```python
from build123d import *

# Parameters (mm, degrees)
SKETCH1_R                               = 75
BOSS_EXTRUDE1_DEPTH                     = 10
SKETCH3_R                               = 4.5
CUT_EXTRUDE2_DEPTH                      = 10
SKETCH5_W                               = 2.667
SKETCH5_H                               = 4.572
SKETCH6_R                               = 55
SKETCH6_R_2                             = 53
CUT_EXTRUDE3_DEPTH                      = 1.3208
SKETCH10_R                              = 2
CUT_EXTRUDE6_DEPTH                      = 11
CBORE_FOR_M5_HEX_HEAD_BOLT1_D           = 5.5
CBORE_FOR_M5_HEX_HEAD_BOLT1_CBORE_D     = 12.238
CBORE_FOR_M5_HEX_HEAD_BOLT1_CBORE_DEPTH = 3.5
SKETCH16_R                              = 75
SKETCH16_R_2                            = 68
CUT_EXTRUDE10_DEPTH                     = 10
CIRPATTERN1_COUNT                       = 12
CIRPATTERN2_COUNT                       = 8
SKETCH17_R                              = 6.119
CUT_EXTRUDE11_DEPTH                     = 5
CIRPATTERN3_COUNT                       = 8
SKETCH18_R                              = 15
CUT_EXTRUDE12_DEPTH                     = 10


with BuildPart() as part:
    # Sketch1 → Boss-Extrude1 (new body)
    with BuildSketch(Plane.XY):
        Circle(SKETCH1_R)
    extrude(amount=BOSS_EXTRUDE1_DEPTH)

    # Sketch3 → Cut-Extrude2 (cut)
    with BuildSketch(Plane.XY.offset(10)):
        Circle(SKETCH3_R)
    extrude(amount=-CUT_EXTRUDE2_DEPTH, mode=Mode.SUBTRACT)

    # Sketch5 → Cut-Revolve1 (revolve, cut)
    with BuildSketch(Plane(origin=(0, 0, 0), x_dir=(0, 0, -1), z_dir=(1, 0, 0))):
        with Locations((-1.3335, 24.8666)):
            Rectangle(SKETCH5_W, SKETCH5_H)
    revolve(axis=Axis((0, 0, 0), (0, 0, -1)), mode=Mode.SUBTRACT)

    # Sketch6 → Cut-Extrude3 (cut)
    with BuildSketch(Plane.XY.offset(10)):
        Circle(SKETCH6_R)
        Circle(SKETCH6_R_2, mode=Mode.SUBTRACT)
    extrude(amount=-CUT_EXTRUDE3_DEPTH, mode=Mode.SUBTRACT)

    # Sketch10 → Cut-Extrude6 (cut, through all)
    with BuildSketch(Plane(origin=(0, 0, 0), x_dir=(-1, 0, 0), z_dir=(0, 0, -1))):
        with Locations((0, 61)):
            Circle(SKETCH10_R)
    cut_extrude6 = extrude(amount=-CUT_EXTRUDE6_DEPTH, mode=Mode.SUBTRACT)

    # CBORE for M5 Hex Head Bolt1 (through all)
    with Locations(Plane(origin=(0, 0, 0), x_dir=(-1, 0, 0), z_dir=(0, 0, -1))):
        with Locations((-28.284271247, 28.284271247)):
            cbore_for_m5_hex_head_bolt1 = CounterBoreHole(CBORE_FOR_M5_HEX_HEAD_BOLT1_D / 2, CBORE_FOR_M5_HEX_HEAD_BOLT1_CBORE_D / 2, CBORE_FOR_M5_HEX_HEAD_BOLT1_CBORE_DEPTH)

    # Sketch16 → Cut-Extrude10 (cut)
    with BuildSketch(Plane(origin=(0, 0, 0), x_dir=(-1, 0, 0), z_dir=(0, 0, -1))):
        Circle(SKETCH16_R)
        Circle(SKETCH16_R_2, mode=Mode.SUBTRACT)
    extrude(amount=-CUT_EXTRUDE10_DEPTH, mode=Mode.SUBTRACT)

    # CirPattern1: Cut-Extrude6 ×12 about axis
    cirpattern1_axis = Axis((0, 0, 0), (0, 0, 1))
    for i in range(1, CIRPATTERN1_COUNT):
        add(cut_extrude6.rotate(cirpattern1_axis, i * 360 / CIRPATTERN1_COUNT), mode=Mode.SUBTRACT)

    # CirPattern2: CBORE for M5 Hex Head Bolt1 ×8 about axis
    cirpattern2_axis = Axis((0, 0, 0), (0, 0, 1))
    for i in range(1, CIRPATTERN2_COUNT):
        add(cbore_for_m5_hex_head_bolt1.rotate(cirpattern2_axis, i * 360 / CIRPATTERN2_COUNT), mode=Mode.SUBTRACT)

    # Sketch17 → Cut-Extrude11 (cut)
    with BuildSketch(Plane(origin=(0, 0, 0), x_dir=(-1, 0, 0), z_dir=(0, 0, -1))):
        with Locations((-28.284271247, 28.284271247)):
            Circle(SKETCH17_R)
    cut_extrude11 = extrude(amount=-CUT_EXTRUDE11_DEPTH, mode=Mode.SUBTRACT)

    # CirPattern3: Cut-Extrude11 ×8 about axis
    cirpattern3_axis = Axis((0, 0, 0), (0, 0, -1))
    for i in range(1, CIRPATTERN3_COUNT):
        add(cut_extrude11.rotate(cirpattern3_axis, i * 360 / CIRPATTERN3_COUNT), mode=Mode.SUBTRACT)

    # Sketch18 → Cut-Extrude12 (cut)
    with BuildSketch(Plane(origin=(0, 0, 0), x_dir=(-1, 0, 0), z_dir=(0, 0, -1))):
        Circle(SKETCH18_R)
    extrude(amount=-CUT_EXTRUDE12_DEPTH, mode=Mode.SUBTRACT)


solid = part.part
```
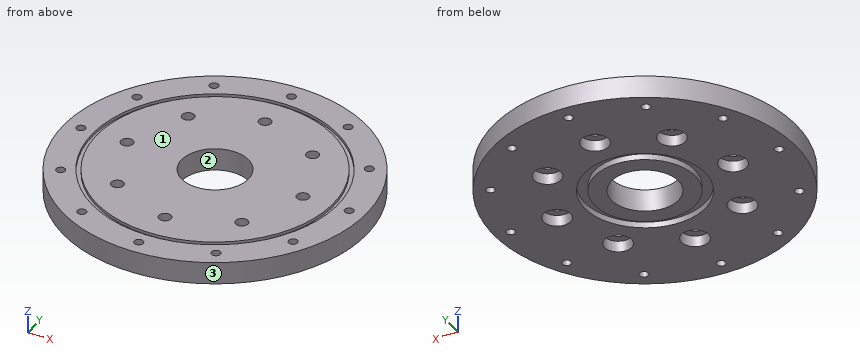
Here's how the part is built. I have some questions about the finished solid (model axes, mm). Face numbers are marked on the shaded views. Round coordinates to 2 decimals unless told otherwise and drop trailing zeros. Loops run counter-clockwise (first coordinate to the right, second up) from the corner with the lowest first, then second, coordinate; pieces in that order, holes last. Notation, with made-up numbers: (13.25, 42) -> (24.25, 42) arc R32 cw to (24.25, 73) -> close; hole circle Ø3 at (20.5, -24). An arc over 180 degrees is marked (long way). Answer as CSV lines item,"result". Start each with the question number.
1. I need wall thicknesses on probe 1 along Y at (x, z) = (0, 5.25); probe 2 along Y at (x, z) = (-40, 6.2). Which ranges of each line are inside material? Lowest first, please. Write a range as from..to.
2. I'm going to push flat-ended pins straight in: P1, Ø6, axis at y = -41, z = 5, coming from the -X side; P2, Ø6.5, axis at x = 0, y = -40, coming from the -Z side; P3, Ø2, axis at y = -15.5, z = 4, coming from the -X side. Where does each tip first touch, or does it pass through?
3. If we mould it in two halves opening along Y, with no side actions, what happens to the marked faces 1, 2 and 3? For each: pulls with the +Y half, pulls with the -Y half, needs draft (parallel to the pull), parting line crosses it, or undercut.
4. Imagine slicing it at A-A on y = -61. Write out the boundary of the cut face in (x, z).
5. Imagine slicing it at B-B on x = -40. Write out the boundary of the cut face in (y, z).
Solution:
1,probe 1,"-68..-63, -59..-42.75, -37.25..-15, 15..37.25, 42.75..59, 63..68"
1,probe 2,"-54.99..-2.75, 2.75..54.99"
2,P1,"x = -56.39"
2,P2,"z = 5"
2,P3,"x = -66.44"
3,face 1,"needs draft"
3,face 2,"undercut"
3,face 3,"parting line crosses it"
4,outline,"(-30.05, 0) -> (-2, 0) -> (-2, 10) -> (-30.05, 10) -> close; (2, 0) -> (30.05, 0) -> (30.05, 10) -> (2, 10) -> close"
5,outline,"(-54.99, 0) -> (-6.12, 0) -> (-6.12, 5) -> (-2.75, 5) -> (-2.75, 10) -> (-34.77, 10) -> (-34.77, 8.68) -> (-37.75, 8.68) -> (-37.75, 10) -> (-54.99, 10) -> close; (2.75, 5) -> (6.12, 5) -> (6.12, 0) -> (54.99, 0) -> (54.99, 10) -> (37.75, 10) -> (37.75, 8.68) -> (34.77, 8.68) -> (34.77, 10) -> (2.75, 10) -> close"
